Source: CAD feature listing. Evaluate the final solid. Frame: model axes, mm. Give positions to 0.01 mm unless a question says otherwise; leave off trailing zeros. Loops run counter-clockwise (first coordinate to the right, second up) from the corner with the lowest first, then second, coordinate; pieces in that order, holes last. Notation, with made-up numbers: (34.5, 73) - (39.5, 73) arc R30 cw to (39.5, 109) - close; hole circle Ø6 at (15, 65.25). An arc over 180 degrees is marked (long way). Put each result on its own line as item: value.
```python
from build123d import *

# Parameters (mm, degrees)
F0_W     = 82.946875
F0_H     = 25.908
F0_R     = 3.3734375
F0_R_2   = 9.779
F1_DEPTH = 6.35
F2_R     = 0.889
F3_DEPTH = 3.2164930276
F4_R     = 5.08
F5_SIZE  = 0.508


with BuildPart() as f1:
    # F0 (on Top) → F1 (new body)
    with BuildSketch(Plane.XY):
        Rectangle(F0_W, F0_H)
        with Locations((-31.75, 0)):
            Circle(F0_R, mode=Mode.SUBTRACT)
        Circle(F0_R_2, mode=Mode.SUBTRACT)
        with Locations((31.75, 0)):
            Circle(F0_R, mode=Mode.SUBTRACT)
    extrude(amount=F1_DEPTH)

    # F2 (on face) → F3 (cut, through all)
    with BuildSketch(Plane.XZ.offset(12.954)):
        with Locations((0, 3.175)):
            Circle(F2_R)
    extrude(amount=-F3_DEPTH, mode=Mode.SUBTRACT)

    # F4
    f4_edges = [f1.edges().sort_by_distance(p)[0] for p in [
        (41.473438, -12.954, 3.175),
        (41.473438, 12.954, 3.175),
        (-41.473438, -12.954, 3.175),
        (-41.473438, 12.954, 3.175),
    ]]
    fillet(f4_edges, radius=F4_R)

    # F5
    f5_edges = [f1.edges().sort_by_distance(p)[0] for p in [
        (-35.123438, 0, 6.35),
        (28.376562, 0, 6.35),
    ]]
    chamfer(f5_edges, length=F5_SIZE)


solid = f1.part
```
1) Section query A-A, the plane x = 31.75. Output: boundary loops of the cut face in (y, z).
Check result:
outline: (-12.95, 0) - (-3.37, 0) - (-3.37, 5.84) - (-3.88, 6.35) - (-12.95, 6.35) - close; (3.37, 0) - (12.95, 0) - (12.95, 6.35) - (3.88, 6.35) - (3.37, 5.84) - close
2) Section query C-C, the plane y = 0. Output: boundary loops of the cut face in (x, z).
Check result:
outline: (-41.47, 0) - (-35.12, 0) - (-35.12, 5.84) - (-35.63, 6.35) - (-41.47, 6.35) - close; (-28.38, 0) - (-9.78, 0) - (-9.78, 6.35) - (-27.87, 6.35) - (-28.38, 5.84) - close; (9.78, 0) - (28.38, 0) - (28.38, 5.84) - (27.87, 6.35) - (9.78, 6.35) - close; (35.12, 0) - (41.47, 0) - (41.47, 6.35) - (35.63, 6.35) - (35.12, 5.84) - close
3) Pin query (flat end, axial travel): P1, Ø1.1, axis at x = 0, z = 3.175, coming from the -Y side; P2, Ø5.5, axis at x = 31.75, y = 0, coming from the -Z side. Return the tip coordinate at first contact, or that it passes through.
Check result:
P1: y = 9.76
P2: through
4) Section query B-B, the plane z = 5. Output: boundary loops of the cut face in (x, y).
Check result:
outline: (-41.47, -7.87) arc R5.08 ccw to (-36.39, -12.95) - (36.39, -12.95) arc R5.08 ccw to (41.47, -7.87) - (41.47, 7.87) arc R5.08 ccw to (36.39, 12.95) - (-36.39, 12.95) arc R5.08 ccw to (-41.47, 7.87) - close; hole circle Ø6.75 at (-31.75, 0); hole circle Ø19.56 at (0, 0); hole circle Ø6.75 at (31.75, 0)
5) Section query D-D, the plane x = 0. Output: boundary loops of the cut face in (y, z).
Check result:
outline: (-12.95, 0) - (-9.78, 0) - (-9.78, 2.29) - (-12.95, 2.29) - close; (-12.95, 4.06) - (-9.78, 4.06) - (-9.78, 6.35) - (-12.95, 6.35) - close; (9.78, 0) - (12.95, 0) - (12.95, 6.35) - (9.78, 6.35) - close
6) Material intervals for line 1 along X through (y, z) = (-0.25, 1.75); line 2 along X through (y, z) = (-0.75, 2); line 3 along Y through (x, z) = (-31.5, 5.5), sorted ascending. Write a range as [from, to].
Check result:
line 1: [-41.47, -35.11], [-28.39, -9.78], [9.78, 28.39], [35.11, 41.47]
line 2: [-41.47, -35.04], [-28.46, -9.75], [9.75, 28.46], [35.04, 41.47]
line 3: [-12.95, -3.36], [3.36, 12.95]
7) Mould query, pull axis Z, two halves, no side actions, for faces 1 (the flat face through (-10, 0, 0)), 2 (the cylindrical face through (0.478, -11.369, 3.925)), 3 (the cylindrical face through (28.38, 0.15, 2.88)). Classes: pulls with the +Z half, pulls with the -Z half, needs draft (parallel to the pull), parting line crosses it, or undercut.
Check result:
face 1: pulls with the -Z half
face 2: undercut
face 3: needs draft
